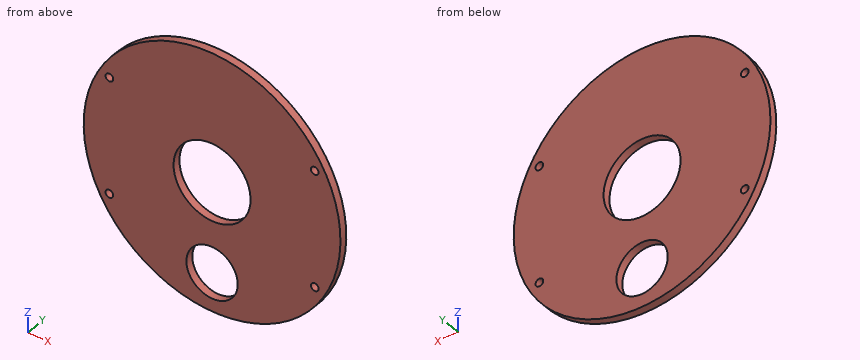
```python
from build123d import *

# Parameters (mm, degrees)
SKETCH1_R           = 50
SKETCH1_R_2         = 1.5
BOSS_EXTRUDE1_DEPTH = 3
SKETCH2_R           = 15
CUT_EXTRUDE1_DEPTH  = 10
SKETCH3_R           = 10
CUT_EXTRUDE2_DEPTH  = 10


with BuildPart() as part:
    # Sketch1 → Boss-Extrude1 (new body)
    with BuildSketch(Plane(origin=(0, 0, 0), x_dir=(1, 0, 0), z_dir=(0, 1, 0))):
        with Locations(Location((0, 0, 0), (0, 0, 270))):
            Circle(SKETCH1_R)
        with Locations(Location((-40, 22.5, 0), (0, 0, 270))):
            Circle(SKETCH1_R_2, mode=Mode.SUBTRACT)
        with Locations(Location((40, 22.5, 0), (0, 0, 270))):
            Circle(SKETCH1_R_2, mode=Mode.SUBTRACT)
        with Locations(Location((40, -22.5, 0), (0, 0, 270))):
            Circle(SKETCH1_R_2, mode=Mode.SUBTRACT)
        with Locations(Location((-40, -22.5, 0), (0, 0, 270))):
            Circle(SKETCH1_R_2, mode=Mode.SUBTRACT)
    extrude(amount=BOSS_EXTRUDE1_DEPTH)

    # Sketch2 → Cut-Extrude1 (cut)
    with BuildSketch(Plane(origin=(0, 3, 0), x_dir=(1, 0, 0), z_dir=(0, 1, 0))):
        with Locations(Location((0, 0, 0), (0, 0, 270))):
            Circle(SKETCH2_R)
    extrude(amount=-CUT_EXTRUDE1_DEPTH, mode=Mode.SUBTRACT)

    # Sketch3 → Cut-Extrude2 (cut)
    with BuildSketch(Plane.XZ):
        with Locations(Location((0, -35, 0), (0, 0, 270))):
            Circle(SKETCH3_R)
    extrude(amount=-CUT_EXTRUDE2_DEPTH, mode=Mode.SUBTRACT)


solid = part.part
```
Can you work these out from the model? Positions are in its coordinate system, mm. Round coordinates to 2 decimals unless told otherwise and drop trailing zeros. Loops run counter-clockwise (first coordinate to the right, second up) from the corner with the lowest first, then second, coordinate; pieces in that order, holes last. Notation, with made-up numbers: M -20,84.5 L 1,84.5 A18 cw 1,115.5 Z; hole C -20,62.25 d8. An arc over 180 degrees is marked long. Write item = value, one per line. Start each with the question number.
(1) Suppose I cut it at A-A on x = 40. Write out the boundary of the cut face in (y, z), plus the area to 3 significant figures.
(2) Suppose I cut it at B-B on y = 0.9. Write out the boundary of the cut face in (x, z), plus the area to 3 significant figures.
(3) I need wall thicknesses on line 1 along X through (y, z) = (1.6, 22.5); line 2 along Z through (x, y) = (-3, 1.5); line 3 along Z through (x, y) = (-6, 1.4). Which ranges of each line are inside material? Lowest first, please.
(4) Suppose I cut it at D-D on x = -12.5. Write out the boundary of the cut face in (y, z).
(5) Suppose I cut it at C-C on z = -34.5. Write out the boundary of the cut face in (x, y).
(6) I'm going to push flat-ended pins straight in: P1, Ø4, axis at x = -17.5, z = 36.5, coming from the -Y side; P2, Ø2.5, axis at x = -40, z = 22.5, coming from the +Y side. Where does each tip first touch, or does it pass through?
Answer block:
q1.outline = M 0,-30 L 3,-30 L 3,-24 L 0,-24 Z; M 0,-21 L 3,-21 L 3,21 L 0,21 Z; M 0,24 L 3,24 L 3,30 L 0,30 Z
q1.area = 162 mm²
q2.outline = C 0,0 d100; hole C -40,-22.5 d3; hole C -40,22.5 d3; hole C 0,0 d30; hole C 0,-35 d20; hole C 40,-22.5 d3; hole C 40,22.5 d3
q2.area = 6,800 mm²
q3.line_1 = -44.65 to -41.5, -38.5 to 38.5, 41.5 to 44.65
q3.line_2 = -49.91 to -44.54, -25.46 to -14.7, 14.7 to 49.91
q3.line_3 = -49.64 to -43, -27 to -13.75, 13.75 to 49.64
q4.outline = M 0,-48.41 L 3,-48.41 L 3,-8.29 L 0,-8.29 Z; M 0,8.29 L 3,8.29 L 3,48.41 L 0,48.41 Z
q5.outline = M -36.19,0 L -9.99,0 L -9.99,3 L -36.19,3 Z; M 9.99,0 L 36.19,0 L 36.19,3 L 9.99,3 Z
q6.P1 = 0
q6.P2 = through
